from build123d import *

# Parameters (mm, degrees)
SKETCH1_R                = 25.35
SKETCH1_R_2              = 19
BOSS_EXTRUDE1_DEPTH      = 12.7
BODY_DELETE_KEEP_1_DEPTH = 12.7
SKETCH2_W                = 15.24
SKETCH2_H                = 12.7
SKETCH2_R                = 2.5
BOSS_EXTRUDE2_DEPTH      = 5.08


# Read off the part's stored shape, not the designer's step: Body-Delete/Keep 1
with BuildPart() as part:
    # Sketch1 → Boss-Extrude1 (new body)
    with BuildSketch(Plane.XY):
        Circle(SKETCH1_R)
        Circle(SKETCH1_R_2, mode=Mode.SUBTRACT)
    extrude(amount=BOSS_EXTRUDE1_DEPTH)


with BuildPart() as body_2:
    # Split1: the piece on the far side of the plane
    add(part.part)
    split(bisect_by=Plane.ZX, keep=Keep.BOTTOM)

    # Body-Delete/Keep 1 outline → Body-Delete/Keep 1 (cut)
    with BuildSketch(Plane.XY):
        with BuildLine():
            ThreePointArc((-25.35, 0), (0, -25.35), (25.35, 0))
            Line((25.35, 0), (19, 0))
            ThreePointArc((19, 0), (0, -19), (-19, 0))
            Line((-19, 0), (-25.35, 0))
        make_face()
    extrude(amount=BODY_DELETE_KEEP_1_DEPTH, mode=Mode.SUBTRACT)


with BuildPart() as part_1:
    add(part.part)

    # Split1
    split(bisect_by=Plane.ZX, keep=Keep.TOP)

    # Sketch2 → Boss-Extrude2 (add)
    # profile 1 of 2: a face of its own
    with BuildSketch(Plane.XZ):
        with Locations((26.62, 6.35)):
            Rectangle(SKETCH2_W, SKETCH2_H)
        with Locations(Location((30.43, 6.35, 0), (0, 0, 270))):
            Circle(SKETCH2_R, mode=Mode.SUBTRACT)
    # profile 2 of 2: a face of its own
    with BuildSketch(Plane.XZ):
        with Locations((-26.62, 6.35)):
            Rectangle(SKETCH2_W, SKETCH2_H)
        with Locations(Location((-30.43, 6.35, 0), (0, 0, 90))):
            Circle(SKETCH2_R, mode=Mode.SUBTRACT)
    extrude(amount=-BOSS_EXTRUDE2_DEPTH)


solid = part_1.part
Source: CAD feature listing. Evaluate the final solid. Frame: model axes, mm. A direction names the side the tool comes from. Round coordinates to 2 decimals unless told otherwise and drop trailing zeros. Loops run counter-clockwise (first coordinate to the right, second up) from the corner with the lowest first, then second, coordinate; pieces in that order, holes last. Notation, with made-up numbers: (49.25, 32.5) -> (101.25, 32.5) arc R26 cw to (101.25, 46.5) -> close; hole circle Ø7 at (25, -30). An arc over 180 degrees is marked (long way). Answer as a JSON object with one key per item and string values. Group by question number.
Q1. Section query C-C (y = 9.5). Output: boundary loops of the cut face in (x, z).
Q2. Mould query, pull axis X, two halves, no side actions, for faces 4 (the cylindrical face through (27.99, 2.5, 6.89)), 5 (the cylindrical face through (-27.99, 2.5, 5.81)), 6 (the flat face through (-34.24, 3, 6)), 7 (the flat face through (-27, 0, 6)). Classes: pulls with the +X half, pulls with the -X half, needs draft (parallel to the pull), parting line crosses it, or undercut.
Q3. Section query D-D (z = 1.25). Output: boundary loops of the cut face in (x, y).
Q4. Section query A-A (x = -30.43). Output: boundary loops of the cut face in (y, z).
Q5. Section query B-B (z = 6.35). Output: boundary loops of the cut face in (x, y).
Q6. Ray query, line 1 (X direction, y = 2, z = 8); line 2 (X direction, y = 1.25, z = 6.35); line 3 (X direction, y = 9, z = 7.25). Return the intervals inside material, ascending. Write a range as from..to.
Q7. Contact query for flat-ended pins moving along their axis: P1, Ø4, axis at x = 11, z = 2, coming from the -Y side; P2, Ø3, axis at x = -27.5, z = 4, coming from the +Y side; P3, Ø2, axis at x = -12.5, z = 9.5, coming from the -Y side; P4, Ø4, axis at x = -30.43, z = 6.35, coming from the +Y side. Output: stop coordinate, or through.
Q8. Access query for faces 1 (the flat face through (28, 5.08, 8)), 2 (the flat face through (-27.5, 5.08, 6.4)), 3 (the cylindrical face through (0.486, 25.345, 6.261)). Directions: +Z, -Z, +X, -X, +Y, -Y. A direction counts if a zero-diameter tool reaches every point of the face in a straight line with its end or side. Return the directions, or none.
Completed:
{
 "1": {"outline": "(-23.5, 0) -> (-16.45, 0) -> (-16.45, 12.7) -> (-23.5, 12.7) -> close; (16.45, 0) -> (23.5, 0) -> (23.5, 12.7) -> (16.45, 12.7) -> close"},
 "2": {"face 4": "undercut", "face 5": "undercut", "face 6": "pulls with the -X half", "face 7": "needs draft"},
 "3": {"outline": "(-34.24, 0) -> (-19, 0) arc R19 cw to (19, 0) -> (34.24, 0) -> (34.24, 5.08) -> (24.84, 5.08) arc R25.35 ccw to (-24.84, 5.08) -> (-34.24, 5.08) -> close"},
 "4": {"outline": "(0, 0) -> (5.08, 0) -> (5.08, 3.85) -> (0, 3.85) -> close; (0, 8.85) -> (5.08, 8.85) -> (5.08, 12.7) -> (0, 12.7) -> close"},
 "5": {"outline": "(-34.24, 0) -> (-32.93, 0) -> (-32.93, 5.08) -> (-34.24, 5.08) -> close; (-27.93, 0) -> (-19, 0) arc R19 cw to (19, 0) -> (27.93, 0) -> (27.93, 5.08) -> (24.84, 5.08) arc R25.35 ccw to (-24.84, 5.08) -> (-27.93, 5.08) -> close; (32.93, 0) -> (34.24, 0) -> (34.24, 5.08) -> (32.93, 5.08) -> close"},
 "6": {"line 1": "-34.24..-32.31, -28.55..-18.89, 18.89..28.55, 32.31..34.24", "line 2": "-34.24..-32.93, -27.93..-18.96, 18.96..27.93, 32.93..34.24", "line 3": "-23.7..-16.73, 16.73..23.7"},
 "7": {"P1": "y = 13.86", "P2": "y = 5.08", "P3": "y = 13.37", "P4": "through"},
 "8": {"face 1": "+Z, -Z, +X, +Y", "face 2": "+Z, -Z, -X, +Y", "face 3": "+Z, -Z, +Y"}
}
